For this review, take the finished solid that the model builds, in its own axes (mm). Give positions to 0.01 mm unless a question says otherwise; leave off trailing zeros. Write each loop counter-clockwise with the first axis right and the second up, starting at its lowest first coordinate (ties: lowest second). Pieces come first, ordered by that corner, then holes.
Q1. We need section A-A (z = -147.5). Write out the cut boundary in (x, y), then the cut area to 3 significant figures.
Q2. Mouldability with a two-part tool opening along Z and no side actions: class faces 1 (the flat face through (-10, 0, -79)), 2 (the flat face through (-12, 3, 0)), 3 (the cylindrical face through (-10.06, 2.96, -13.04)) as released by +Z, released by -Z, zero draft, split by the parting line, or undercut.
Q3. Insertion check: P1, Ø4.5, axis at x = -12.5, z = -12.5, coming from the -Y side. The pin has a flat end and moves straight along its axis. Give the tip position at first contact, or say it passes through.
Q4. For line 1 (Z direction, x = -12.5, y = 2.8); line 2 (X direction, y = 2.8, z = -147.5); line 3 (Z direction, x = -10.5, y = 5.45), list the stretches that pass through material, from the lowest coordinate up.
Autodesk Inventor part; units mm, degrees
ref_plane "YZ Plane" through (0, 0, 0) normal (1, 0, 0) x (0, 1, 0)
ref_plane "XZ Plane" through (0, 0, 0) normal (0, 1, 0) x (-1, 0, 0)
ref_plane "XY Plane" through (0, 0, 0) normal (0, 0, 1) x (1, 0, 0)
sketch "Sketch1" plane through (0, 0, 0) normal (0, 1, 0) x (-1, 0, 0)
  line L0 (0, 0) -> (25, 0)
  line L1 (25, 0) -> (25, -160)
  line L2 (25, -160) -> (0, -160)
  line L3 (0, -160) -> (0, 0)
  dimension "d0" = 25
  dimension "d1" = 160
extrude "Extrusion1" add sketch "Sketch1" along normal blind 6
sketch "Sketch2" plane through (0, 6, 0) normal (0, 1, 0) x (1, 0, 0)
  line L0 (-25, 160) -> (-25, 0)
  line L1 (-25, 0) -> (0, 0)
  line L2 (0, 160) -> (-25, 160)
  point P0 (-12.5, 12.5)
  point P1 (-12.5, 147.5)
  dimension "d4" = 25
  dimension "d5" = 160
  dimension "d6" = 12.5
  dimension "d7" = 12.5
  dimension "d8" = 12.5
  dimension "d9" = 12.5
hole "Hole1" at (-12.5, 6, -12.5) at (-12.5, 6, -147.5) direction (0, -1, 0) diameter 5 end through all
sketch "Esboço3" plane through (0, 6, 0) normal (0, 1, 0) x (1, 0, 0)
  line L0 (0, 160) -> (-25, 160)
  line L1 (0, 0) -> (0, 160)
  line L2 (-25, 160) -> (-25, 0)
  line L3 (-25, 0) -> (0, 0)
  point P0 (-12.5, 80)
  point P1 (-12.5, 0)
  dimension "d17" = 160
  dimension "d18" = 25
  dimension "d19" = 12.5
  dimension "d20" = 80
hole "Furo2" at (-12.5, 6, -80) direction (0, -1, 0) diameter 5 depth 6
thread "Rosca1"
thread "Rosca2"
equation "\"d15\" = Thickness"
equation "\"d26\" = Thickness"
equation "\"BendRadius\" = Thickness"
equation "\"BendReliefWidth\" = Thickness"
equation "\"BendReliefDepth\" = 0.5 * Thickness"
equation "\"CornerReliefSize\" = 4 * Thickness"
equation "\"MinimumRemnant\" = 2 * Thickness"
equation "\"TransitionRadius\" = BendRadius"
equation "\"JacobiRadiusSize\" = BendRadius"
equation "\"GapSize\" = Thickness"
properties part number "Suporte mesa" material "Aluminum 6061"
Computed:
1. outline: (-25, 0) - (-15, 0) - (-15, 6) - (-25, 6) - close; (-10, 0) - (0, 0) - (0, 6) - (-10, 6) - close
1. area: 120 mm2
2. face 1: zero draft
2. face 2: released by +Z
2. face 3: undercut
3. P1: passes through
4. line 1: z = -160 to -150, -145 to -82.5, -77.5 to -15, -10 to 0
4. line 2: x = -25 to -15, -10 to 0
4. line 3: z = -160 to -149, -146 to -81.5, -78.5 to -14, -11 to 0
